```python
from build123d import *

# Parameters (mm, degrees)
F0_W     = 90
F0_H     = 30
F1_DEPTH = 1
F2_R     = 1
F3_DEPTH = 1
F4_SIZE  = 2
F5_R     = 1.5
F6_DEPTH = 1


with BuildPart() as f1:
    # F0 (on Top) → F1 (new body)
    with BuildSketch(Plane.XY):
        with Locations((45, 15)):
            Rectangle(F0_W, F0_H)
    extrude(amount=F1_DEPTH)

    # F2 (on Top) → F3 (cut, through all)
    with BuildSketch(Plane.XY):
        with Locations((12.444126, 6)):
            Circle(F2_R)
        with Locations((12.444126, 21)):
            Circle(F2_R)
        with Locations((12.444126, 16)):
            Circle(F2_R)
        with Locations((21.444126, 21)):
            Circle(F2_R)
        with Locations((21.444126, 16)):
            Circle(F2_R)
        with Locations((21.444126, 6)):
            Circle(F2_R)
        with Locations((30.444126, 21)):
            Circle(F2_R)
        with Locations((30.444126, 16)):
            Circle(F2_R)
        with Locations((30.444126, 6)):
            Circle(F2_R)
        with Locations((39.444126, 21)):
            Circle(F2_R)
        with Locations((39.444126, 16)):
            Circle(F2_R)
        with Locations((39.444126, 6)):
            Circle(F2_R)
        with Locations((48.444126, 21)):
            Circle(F2_R)
        with Locations((48.444126, 16)):
            Circle(F2_R)
        with Locations((48.444126, 6)):
            Circle(F2_R)
        with Locations((57.444126, 21)):
            Circle(F2_R)
        with Locations((57.444126, 16)):
            Circle(F2_R)
        with Locations((57.444126, 6)):
            Circle(F2_R)
        with Locations((66.444126, 21)):
            Circle(F2_R)
        with Locations((66.444126, 16)):
            Circle(F2_R)
        with Locations((66.444126, 6)):
            Circle(F2_R)
        with Locations((75.444126, 21)):
            Circle(F2_R)
        with Locations((75.444126, 16)):
            Circle(F2_R)
        with Locations((75.444126, 6)):
            Circle(F2_R)
    extrude(amount=F3_DEPTH, mode=Mode.SUBTRACT)

    # F4
    f4_edges = [f1.edges().sort_by_distance(p)[0] for p in [
        (90, 0, 0.5),
    ]]
    chamfer(f4_edges, length=F4_SIZE)

    # F5 (on Top) → F6 (cut, through all)
    with BuildSketch(Plane.XY):
        with Locations((5, 6)):
            Circle(F5_R)
        with Locations((5, 21)):
            Circle(F5_R)
        with Locations((85, 21)):
            Circle(F5_R)
        with Locations((85, 6)):
            Circle(F5_R)
    extrude(amount=F6_DEPTH, mode=Mode.SUBTRACT)


solid = f1.part
```
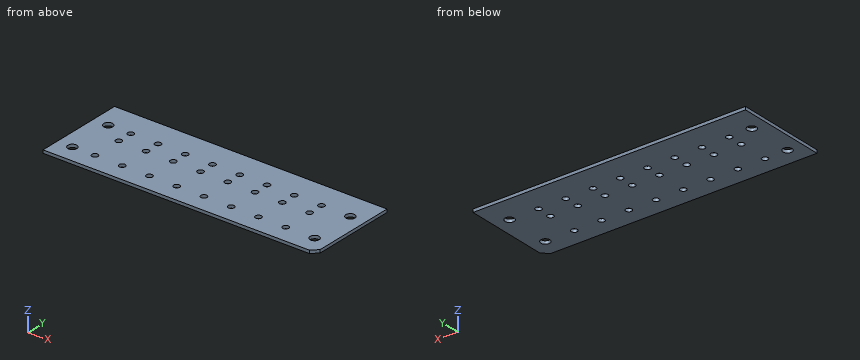
The model under review builds one solid part; all positions refer to its coordinate system, in mm. Round coordinates to 2 decimals unless told otherwise and drop trailing zeros. Loops run counter-clockwise (first coordinate to the right, second up) from the corner with the lowest first, then second, coordinate; pieces in that order, holes last. Notation, with made-up numbers: (67, 40.25) - (104, 40.25) arc R33 ccw to (104, 72.25) - close; hole circle Ø5 at (34.5, -22). An arc over 180 degrees is marked (long way). Write each question's results on one line, items separated by ' | '. Start each with the question number.
Q1. Take a section at B-B on z = 0.5. Give the number of separate pieces and of enclosed holes in the cut face, plus the area to 3 significant figures.
Q2. Insertion check: P1, Ø2.5, axis at x = 48.44, y = 16, coming from the -Z side. The pin has a flat end and moves straight along its axis. Give the tip position at first contact, or say it passes through.
Q3. Wall thickness on line 1 along Y through (x, z) = (5, 0.65); line 2 along Y through (x, z) = (13, 0.2); line 3 along Y through (x, z) = (12, 0.5): over which ranges is each line inside the solid? List them lowest first. Write a range as [from, to].
Q4. Take a section at A-A on x = 85. Give the boundary of the cut face in (y, z).
Data:
1) separate pieces: 1 | enclosed holes: 28 | area: 2,590 mm²
2) P1: stops at z = 0
3) line 1: y = [0, 4.5], [7.5, 19.5], [22.5, 30] | line 2: y = [0, 5.17], [6.83, 15.17], [16.83, 20.17], [21.83, 30] | line 3: y = [0, 5.1], [6.9, 15.1], [16.9, 20.1], [21.9, 30]
4) outline: (0, 0) - (4.5, 0) - (4.5, 1) - (0, 1) - close; (7.5, 0) - (19.5, 0) - (19.5, 1) - (7.5, 1) - close; (22.5, 0) - (30, 0) - (30, 1) - (22.5, 1) - close
